```python
from build123d import *

# Parameters (mm, degrees)
F0_W     = 130
F0_H     = 450
F0_R     = 3
F1_DEPTH = 3


with BuildPart() as f1:
    # F0 (on Front) → F1 (new body)
    with BuildSketch(Plane.XZ):
        with Locations((65, 225)):
            Rectangle(F0_W, F0_H)
        with Locations((15, 15)):
            Circle(F0_R, mode=Mode.SUBTRACT)
        with BuildLine():
            ThreePointArc((55, 90), (56.464466, 93.535534), (60, 95))
            Line((60, 95), (85, 95))
            ThreePointArc((85, 95), (88.535534, 93.535534), (90, 90))
            Line((90, 90), (90, 80))
            ThreePointArc((90, 80), (88.535534, 76.464466), (85, 75))
            Line((85, 75), (60, 75))
            ThreePointArc((60, 75), (56.464466, 76.464466), (55, 80))
            Line((55, 80), (55, 90))
        make_face(mode=Mode.SUBTRACT)
        with Locations((115, 15)):
            Circle(F0_R, mode=Mode.SUBTRACT)
        with Locations((15, 435)):
            Circle(F0_R, mode=Mode.SUBTRACT)
        with Locations((115, 435)):
            Circle(F0_R, mode=Mode.SUBTRACT)
    extrude(amount=F1_DEPTH)


solid = f1.part
```
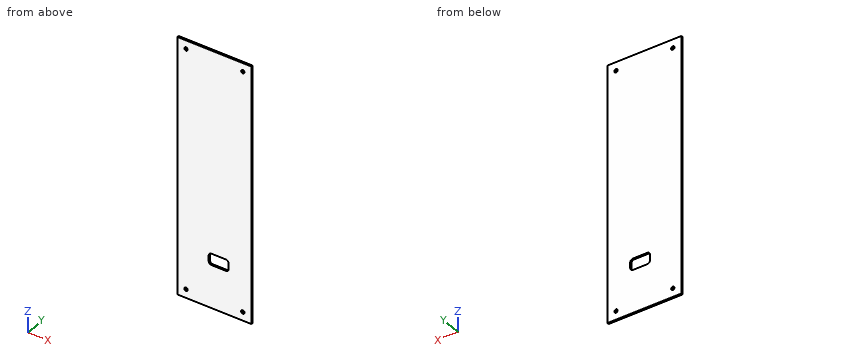
Here's how the part is built. I have some questions about the finished solid (model axes, mm). Round coordinates to 2 decimals unless told otherwise and drop trailing zeros. Loops run counter-clockwise (first coordinate to the right, second up) from the corner with the lowest first, then second, coordinate; pieces in that order, holes last. Notation, with made-up numbers: (11.25, 13) -> (31.25, 13) arc R35 ccw to (31.25, 48) -> close; hole circle Ø8 at (46, 15). An arc over 180 degrees is marked (long way). Answer as CSV lines item,"result". Start each with the question number.
1. Imagine slicing it at A-A on x = 67.5. Write out the boundary of the cut face in (y, z).
2. I need wall thicknesses on probe 1 along X at (y, z) = (-2.15, 435); probe 2 along Z at (x, y) = (15, -0.65); probe 3 along Z at (x, y) = (61, -0.9). Which ranges of each line are inside material? Lowest first, please. Write a range as from..to.
3. I'm going to push a flat-ended pin straight in: P1, Ø3.5, axis at x = 115, z = 15, coming from the +Y side. Where does the tip first touch, or does it pass through?
Solution:
1,outline,"(-3, 0) -> (0, 0) -> (0, 75) -> (-3, 75) -> close; (-3, 95) -> (0, 95) -> (0, 450) -> (-3, 450) -> close"
2,probe 1,"0..12, 18..112, 118..130"
2,probe 2,"0..12, 18..432, 438..450"
2,probe 3,"0..75, 95..450"
3,P1,"through"
